Check sheet for the modelled part. Datum: model origin and axes. Units: mm. Face numbers are marked on the shaded views. A direction names the side the tool comes from. Give positions to 0.01 mm unless a question says otherwise; leave off trailing zeros. Order: outer loops, then holes, each group sorted by start corner. A loop starts at its lowest first (then second) coordinate and runs counter-clockwise, first axis right, second up. Notation, with made-up numbers: (57.25, 11) -> (97.25, 11) arc R22 ccw to (97.25, 37) -> close; hole circle Ø5 at (-2, -20). An arc over 180 degrees is marked (long way). Answer in a Markdown table with one row per item. Add a question column.
(1) Release check for a two-part mould opening along Z. For the marked faces 1, 2 and 3 record: released by +Z, released by -Z, zero draft, split by the parting line, or undercut.
(2) Set-up check for the marked faces 4, 5, 6, 7 and 8: record each of +Z, -Z, +X, -X, +Y, -Y from which the full face is reachable in a straight line by a thin tool's end or side.
(3) Cross-section at C-C (y = 2.5). Record the cut outline in (x, z), then the cut area to 3 significant figures.
(4) Cross-section at A-A (z = 0). Record the cut outline in (x, y), then the cut area to 3 significant figures.
(5) Go/stop test with flat-tipped pins: pin 1 (3 mm diameter, centred on x = 34, y = -10, fed in from +Z); pin 2 (9 mm diameter, centred on y = -9.5, z = 32, fed in from -X); pin 3 (8 mm diameter, centred on x = 60.5, y = 6, fed in from +Z); pin 4 (11.5 mm diameter, centred on x = 63, z = -7.5, fed in from -Y). Record where each tip stops, or that it passes through.
(6) Cross-section at D-D (z = 17). State how many separate pieces and enclosed holes the cut face has, then the cut area to 3 significant figures.
(7) Cross-section at B-B (x = 85). Record the cut outline in (y, z), then the cut area to 3 significant figures.
(8) Thickness scan on L1, parallel to X at y = -8.5, z = 0; L2, parallel to X at y = -8, z = -12; L3, parallel to X at y = 12, z = 28.5. Record the ranges inside material, lowest first. Write a range as [from, to].
```python
from build123d import *

# Parameters (mm, degrees)
F2_DEPTH  = 18
F0_W      = 80
F0_H      = 47.1640562918
F0_H_2    = 42.8359437082
F0_H_3    = 45
F4_DEPTH  = 25
F5_R      = 27.3467975621
F5_R_2    = 27.0757536819
F6_DEPTH  = 58.2
F8_DEPTH  = 18
F9_R      = 25.5810591855
F10_DEPTH = 63.8


# Not quite as in the source:
# - a feature names something its author has since deleted; it is built from what else it names


with BuildPart() as f2:
    # F1 (on face) → F2 (new body)
    with BuildSketch(Plane.XZ):
        Polygon((39.6220497787, 45.2090576291), (-39.5539887249, 45.2090576291), (-40.2230843902, 14.8768285289), (39.6220497787, 14.8768285289), align=None)
    extrude(amount=F2_DEPTH)


with BuildPart() as f2b:
    # F0 (on Front) → F2, piece 2 (new body)
    with BuildSketch(Plane.XZ):
        with Locations((-80, -21.4179718541)):
            Rectangle(F0_W, F0_H)
        Polygon((-40, 2.1640562918), (-40, -45), (40, -45), (40, 0), (40, 45), (-40, 45), align=None)
        with Locations((-80, 23.5820281459)):
            Rectangle(F0_W, F0_H_2)
        with Locations((80, -22.5)):
            Rectangle(F0_W, F0_H_3)
        with Locations((80, 22.5)):
            Rectangle(F0_W, F0_H_3)
    extrude(amount=F2_DEPTH)


with BuildPart() as f4_tool:
    # F3 (on face) → F4 (new body)
    with BuildSketch(Plane.XZ.offset(18)):
        Polygon((39.6220497787, 14.8768285289), (39.6220497787, 45.2090576291), (-39.5539887249, 45.2090576291), (-40.2230843902, 14.8768285289), align=None)
    extrude(amount=-F4_DEPTH)


with BuildPart() as f2_1:
    add(f2.part)

    # F4: cut by f4_tool
    add(f4_tool.part, mode=Mode.SUBTRACT)


with BuildPart() as f2b_1:
    add(f2b.part)

    # F4: cut by f4_tool
    add(f4_tool.part, mode=Mode.SUBTRACT)

    # F5 (on Front) → F6 (cut)
    with BuildSketch(Plane.XZ):
        with Locations((-79.4878825545, 0)):
            Circle(F5_R)
        with Locations((75.41680336, 0)):
            Circle(F5_R_2)
    extrude(amount=F6_DEPTH, mode=Mode.SUBTRACT)

    # F7 (on Front) → F8 (join)
    with BuildSketch(Plane.XZ):
        Polygon((119.3632781506, -45.4373732209), (119.3632781506, 44.861137867), (39.6516397595, 44.9020341039), (39.6516397595, 4.0344810113), (-39.8564524949, 4.0344810113), (-39.8564524949, 44.9020341039), (-120.2343702316, 44.9020341039), (-120.2343702316, -45.4373732209), align=None)
    extrude(amount=-F8_DEPTH)

    # F9 (on Front) → F10 (cut)
    with BuildSketch(Plane.XZ):
        with Locations((79.3142113835, 0)):
            Circle(F9_R)
    extrude(amount=-F10_DEPTH, mode=Mode.SUBTRACT)


solid = f2b_1.part
```
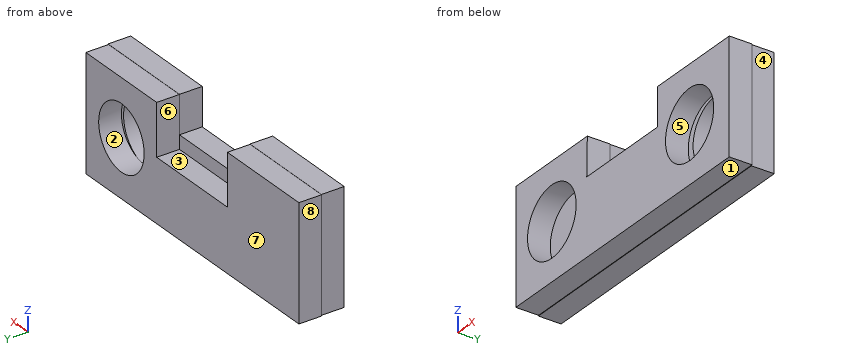
Answer below:
| question | item | result |
|---|---|---|
| 1 | face 1 | released by -Z |
| 1 | face 2 | undercut |
| 1 | face 3 | released by +Z |
| 2 | face 4 | +Z, -Z, +X, +Y |
| 2 | face 5 | -Y |
| 2 | face 6 | +Z, +Y |
| 2 | face 7 | +Z, -Z, +X, -X, +Y |
| 2 | face 8 | +Z, -Z, -X, +Y, -Y |
| 3 | outline | (-120.23, -45.44) -> (119.36, -45.44) -> (119.36, 44.86) -> (39.65, 44.9) -> (39.65, 4.03) -> (-39.86, 4.03) -> (-39.86, 44.9) -> (-120.23, 44.9) -> close; hole circle Ø51.16 at (79.31, 0) |
| 3 | area | 16,300 mm² |
| 4 | outline | (-120.23, 0) -> (-120, 0) -> (-120, -18) -> (-106.83, -18) -> (-106.83, 0) -> (-52.14, 0) -> (-52.14, -18) -> (48.34, -18) -> (48.34, 0) -> (53.73, 0) -> (53.73, 18) -> (-120.23, 18) -> close; (102.49, -18) -> (120, -18) -> (120, 0) -> (119.36, 0) -> (119.36, 18) -> (104.9, 18) -> (104.9, 0) -> (102.49, 0) -> close |
| 4 | area | 5,750 mm² |
| 5 | pin 1 | stops at z = 14.88 |
| 5 | pin 2 | stops at x = -120 |
| 5 | pin 3 | stops at z = 44.89 |
| 5 | pin 4 | passes through |
| 6 | separate pieces | 3 |
| 6 | enclosed holes | 0 |
| 6 | area | 3,550 mm² |
| 7 | outline | (-18, -45) -> (0, -45) -> (0, -45.44) -> (18, -45.44) -> (18, -24.94) -> (0, -24.94) -> (0, -25.32) -> (-18, -25.32) -> close; (-18, 25.32) -> (0, 25.32) -> (0, 24.94) -> (18, 24.94) -> (18, 44.88) -> (0, 44.88) -> (0, 45) -> (-18, 45) -> close |
| 7 | area | 1,440 mm² |
| 8 | L1 | x = [-120, -106.83], [-52.14, 48.34], [102.49, 120] |
| 8 | L2 | x = [-120, -104.06], [-54.91, 51.15], [99.69, 120] |
| 8 | L3 | x = [-120.23, -39.86], [39.65, 119.36] |
